The listing builds one solid part. Answer for the finished solid, in the listing's coordinates (mm). Face numbers are marked on the shaded views. A direction names the side the tool comes from. Round coordinates to 2 decimals unless told otherwise and drop trailing zeros. Write each loop counter-clockwise with the first axis right and the second up, starting at its lowest first coordinate (ties: lowest second). Pieces come first, ordered by that corner, then holes. Notation, with made-up numbers: (32, -5) - (37, -5) arc R30 cw to (37, 17) - close; hole circle Ø9 at (52, -32.75). An arc over 180 degrees is marked (long way). Use a Markdown table: item, result. Add a question column.
1) A cutting plane is placed at A-A (x = -29.5). Give the vertices of the cut face in (y, z), then the cut area to 4 significant figures.
2) Determine the mould class of the marked faces 5, 6 and 7 for opening direction Y: +Y half, -Y half, draft (parallel to the pull), parting line (faces both ways), or undercut.
3) Find the intervals of material crossed by probe 1 along X at (y, z) = (42, 3.5); probe 2 along X at (y, z) = (39, 4.25); probe 3 along Y at (x, z) = (-53, 4.25), in increasing order. Write a range as from..to.
4) A tool of negligible diameter and unlimited length cuts with its end or side. For the marked faces 1, 2, 3 and 4, from which of +Z, -Z, +X, -X, +Y, -Y can it reach the whole face along a straight path? Write none if from no direction.
5) Each of these flat-tipped pins is pushed along its axis until it touches: P1, Ø1.2, axis at x = -34, z = 2.5, coming from the +Y side; P2, Ø1.5, axis at y = 30, z = 4, coming from the +X side; P3, Ø1.5, axis at y = 16.5, z = 4, coming from the -X side. Where does it stop, or does it pass through?
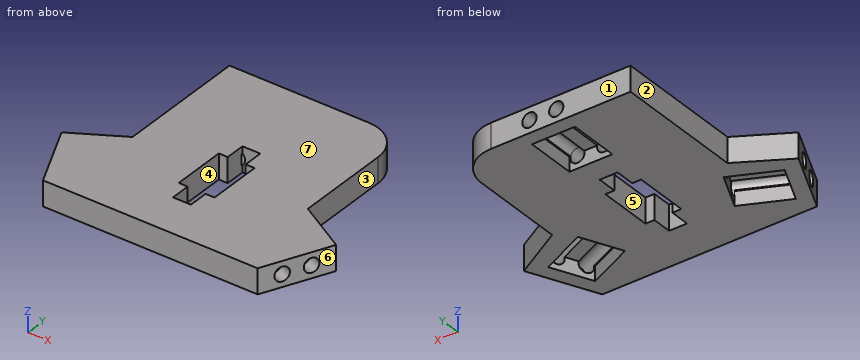
```python
from build123d import *

# Parameters (mm, degrees)
BOSS_EXTRUDE1_DEPTH     = 7
CUT_EXTRUDE1_START      = -25
SKETCH2_R               = 2
CUT_EXTRUDE1_DEPTH      = 26
CUT_EXTRUDE3_DEPTH      = 7
CUT_EXTRUDE2_DEPTH      = 4
CIRPATTERN2_START       = 44.499207337
CIRPATTERN2_DEPTH       = 14
CIRPATTERN2_START_2     = 37.499207337
CIRPATTERN2_2_OUTLINE_R = 2
CIRPATTERN2_2_DEPTH     = 25.000152039
CIRPATTERN2_START_3     = -50.485397831
CIRPATTERN2_3_DEPTH     = 14
CIRPATTERN2_START_4     = -54.485701834
CIRPATTERN2_4_OUTLINE_R = 2
CIRPATTERN2_4_DEPTH     = 25.000304003
FILLET1_R               = 10


# Read off the part's stored shape, not the designer's step: CirPattern2
with BuildPart() as part:
    # Sketch1 → Boss-Extrude1 (new body)
    with BuildSketch(Plane.XY):
        Polygon((-54.5, 62.5), (-5.5, 62.5), (-5.5, 26.172980381), (8.376844495, 18.161180477), (0, 0), (-60, 0), (-68.376844495, 18.161180477), (-54.5, 26.172980381), align=None)
    extrude(amount=BOSS_EXTRUDE1_DEPTH)

    # Sketch2 → Cut-Extrude1 (cut)
    with BuildSketch(Plane(origin=(0, 0, 0), x_dir=(0, 0, -1), z_dir=(0.9080590238365492, -0.41884222474460864, 0)).offset(CUT_EXTRUDE1_START)):
        with Locations(Location((-3.5, 13.75, 0), (0, 0, 270))):
            Circle(SKETCH2_R)
        with Locations(Location((-3.5, 6.25, 0), (0, 0, 270))):
            Circle(SKETCH2_R)
    extrude(amount=CUT_EXTRUDE1_DEPTH, mode=Mode.SUBTRACT)

    # Sketch7 → Cut-Extrude3 (cut)
    with BuildSketch(Plane(origin=(0, 0, 0), x_dir=(-1, 0, 0), z_dir=(0, 0, -1))):
        Polygon((32.5, 17.35), (35, 17.35), (35, 32.35), (32.5, 32.35), (32.5, 37.85), (27.5, 37.85), (27.5, 32.35), (25, 32.35), (25, 17.35), (27.5, 17.35), (27.5, 11.85), (32.5, 11.85), align=None)
    extrude(amount=-CUT_EXTRUDE3_DEPTH, mode=Mode.SUBTRACT)

    # Sketch5 → Cut-Extrude2 (cut)
    with BuildSketch(Plane(origin=(0, 0, 0), x_dir=(-1, 0, 0), z_dir=(0, 0, -1))):
        Polygon((-3.069239501, 16.20431328), (1.956867196, 5.307604994), (14.66969353, 11.171396141), (9.643586833, 22.068104427), align=None)
    extrude(amount=-CUT_EXTRUDE2_DEPTH, mode=Mode.SUBTRACT)

    # CirPattern2 outline → CirPattern2 (cut)
    with BuildSketch(Plane(origin=(0, 0, 0), x_dir=(0.9999999996509443, -2.6421799769471613e-05, 0), z_dir=(2.642179976947161e-05, 0.9999999996509443, 0)).offset(CIRPATTERN2_START)):
        with BuildLine():
            ThreePointArc((-35.687148244, -4), (-33.750656571, -5.5), (-31.814164898, -4))
            Line((-31.814164898, -4), (-28.187148244, -4))
            ThreePointArc((-28.187148244, -4), (-26.250656571, -5.5), (-24.314164898, -4))
            Line((-24.314164898, -4), (-24.000656571, -4))
            Line((-24.000656571, -4), (-24.000656571, 0))
            Line((-24.000656571, 0), (-36.000656571, 0))
            Line((-36.000656571, 0), (-36.000656571, -4))
            Line((-36.000656571, -4), (-35.687148244, -4))
        make_face()
    extrude(amount=CIRPATTERN2_DEPTH, mode=Mode.SUBTRACT)

    # CirPattern2 2 outline → CirPattern2 2 (cut)
    with BuildSketch(Plane(origin=(0, 0, 0), x_dir=(0.9999999996509443, -2.6421799769471613e-05, 0), z_dir=(2.642179976947161e-05, 0.9999999996509443, 0)).offset(CIRPATTERN2_START_2)):
        with Locations((-33.750656571, -3.5)):
            Circle(CIRPATTERN2_2_OUTLINE_R)
        with Locations((-26.250656571, -3.5)):
            Circle(CIRPATTERN2_2_OUTLINE_R)
    extrude(amount=CIRPATTERN2_2_DEPTH, mode=Mode.SUBTRACT)

    # CirPattern2 3 outline → CirPattern2 3 (cut)
    with BuildSketch(Plane(origin=(0, 0, 0), x_dir=(-0.418794239052402, 0.908081155699489, 0), z_dir=(0.908081155699489, 0.418794239052402, 0)).offset(CIRPATTERN2_START_3)):
        with BuildLine():
            ThreePointArc((33.316135564, 4), (31.379643891, 5.5), (29.443152218, 4))
            Line((29.443152218, 4), (29.129643891, 4))
            Line((29.129643891, 4), (29.129643891, 0))
            Line((29.129643891, 0), (41.129643891, 0))
            Line((41.129643891, 0), (41.129643891, 4))
            Line((41.129643891, 4), (40.816135564, 4))
            ThreePointArc((40.816135564, 4), (38.879643891, 5.5), (36.943152218, 4))
            Line((36.943152218, 4), (33.316135564, 4))
        make_face()
    extrude(amount=CIRPATTERN2_3_DEPTH, mode=Mode.SUBTRACT)

    # CirPattern2 4 outline → CirPattern2 4 (cut)
    with BuildSketch(Plane(origin=(0, 0, 0), x_dir=(-0.418794239052402, 0.908081155699489, 0), z_dir=(0.908081155699489, 0.418794239052402, 0)).offset(CIRPATTERN2_START_4)):
        with Locations((31.379643891, 3.5)):
            Circle(CIRPATTERN2_4_OUTLINE_R)
        with Locations((38.879643891, 3.5)):
            Circle(CIRPATTERN2_4_OUTLINE_R)
    extrude(amount=CIRPATTERN2_4_DEPTH, mode=Mode.SUBTRACT)

    # Fillet1
    fillet1_edges = [part.edges().sort_by_distance(p)[0] for p in [
        (-5.5, 62.5, 3.5),
    ]]
    fillet(fillet1_edges, radius=FILLET1_R)


solid = part.part
```
Entries:
| question | item | result |
|---|---|---|
| 1 | outline | (0, 0) - (11.85, 0) - (11.85, 7) - (0, 7) - close; (37.85, 0) - (44.5, 0) - (44.5, 4) - (58.5, 4) - (58.5, 0) - (62.5, 0) - (62.5, 7) - (37.85, 7) - close |
| 1 | area | 199.5 mm² |
| 2 | face 5 | undercut |
| 2 | face 6 | -Y half |
| 2 | face 7 | draft |
| 3 | probe 1 | x = -54.5..-35.75, -31.75..-28.25, -24.25..-5.5 |
| 3 | probe 2 | x = -54.5..-35.6, -31.9..-28.1, -24.4..-5.5 |
| 3 | probe 3 | y = 0..8.07, 12.15..16.33, 20.41..62.5 |
| 4 | face 1 | +Z, -Z, +X, -X, +Y |
| 4 | face 2 | +Z, -Z, -X, +Y |
| 4 | face 3 | +Z, -Z, +X, +Y |
| 4 | face 4 | +Z, -Z |
| 5 | P1 | stops at y = 37.5 |
| 5 | P2 | stops at x = -5.5 |
| 5 | P3 | stops at x = -67.96 |
